from build123d import *

# Parameters (mm, degrees)
SKETCH1_W                                      = 222.53
SKETCH1_H                                      = 135
BOSS_EXTRUDE1_DEPTH                            = 6
FILLET1_R                                      = 5
CSK_FOR_M3_FLAT_HEAD_MACHINE_SCREW1_AT_2_COUNT = 2
CSK_FOR_M3_FLAT_HEAD_MACHINE_SCREW1_AT_2_PITCH = 211.53
CSK_FOR_M3_FLAT_HEAD_MACHINE_SCREW1_AT_3_COUNT = 2
CSK_FOR_M3_FLAT_HEAD_MACHINE_SCREW1_AT_3_PITCH = 245.195719579
CSK_FOR_M3_FLAT_HEAD_MACHINE_SCREW1_AT_4_COUNT = 2
CSK_FOR_M3_FLAT_HEAD_MACHINE_SCREW1_AT_4_PITCH = 124
CHAMFER1_SIZE                                  = 0.5
PCB_CUTOUT_DEPTH                               = 2
SKETCH8_W                                      = 20
SKETCH8_H                                      = 4.7
SKETCH8_W_2                                    = 16
SKETCH8_H_2                                    = 1.6
CABLE_RELIEF_DEPTH                             = 4.5
SKETCH9_W                                      = 25
SKETCH9_H                                      = 25
PI_CUTOUT_DEPTH                                = 3.2
USB_C_CUTOUT_REACH                             = 137
MOUSE_PAD_CUTOUT_DEPTH                         = 1.8
FILLET2_R                                      = 2


with BuildPart() as part:
    # Sketch1 → Boss-Extrude1 (new body)
    with BuildSketch(Plane(origin=(0, 0, 0), x_dir=(1, 0, 0), z_dir=(0, 1, 0))):
        with Locations((111.265, 67.5)):
            Rectangle(SKETCH1_W, SKETCH1_H)
    extrude(amount=BOSS_EXTRUDE1_DEPTH)

    # Fillet1
    fillet1_edges = [part.edges().sort_by_distance(p)[0] for p in [
        (0, 3, -135),
        (222.53, 3, -135),
        (222.53, 3, 0),
        (0, 3, 0),
    ]]
    fillet(fillet1_edges, radius=FILLET1_R)

    # Sketch4 → CSK for M3 Flat Head Machine Screw1 (revolve, cut)
    with BuildSketch(Plane(origin=(5.5, 0, -129.5), x_dir=(0, 0, -1), z_dir=(1, 0, 0))):
        Polygon((0, 0), (0, 6), (1.7, 6), (1.7, 2.95), (3.15, 1.5), (3.15, 0), align=None)
    csk_for_m3_flat_head_machine_screw1 = revolve(axis=Axis((5.5, -6.35, -129.5), (0, 1, 0)), mode=Mode.SUBTRACT)

    # CSK for M3 Flat Head Machine Screw1 at 2: CSK for M3 Flat Head Machine Screw1 ×2
    with Locations(*[(i * CSK_FOR_M3_FLAT_HEAD_MACHINE_SCREW1_AT_2_PITCH, 0, 0) for i in range(1, CSK_FOR_M3_FLAT_HEAD_MACHINE_SCREW1_AT_2_COUNT)]):
        add(csk_for_m3_flat_head_machine_screw1, mode=Mode.SUBTRACT)

    # CSK for M3 Flat Head Machine Screw1 at 3: CSK for M3 Flat Head Machine Screw1 ×2
    with Locations(*[Vector(0.862698584, 0, 0.505718453) * (i * CSK_FOR_M3_FLAT_HEAD_MACHINE_SCREW1_AT_3_PITCH) for i in range(1, CSK_FOR_M3_FLAT_HEAD_MACHINE_SCREW1_AT_3_COUNT)]):
        add(csk_for_m3_flat_head_machine_screw1, mode=Mode.SUBTRACT)

    # CSK for M3 Flat Head Machine Screw1 at 4: CSK for M3 Flat Head Machine Screw1 ×2
    with Locations(*[(0, 0, i * CSK_FOR_M3_FLAT_HEAD_MACHINE_SCREW1_AT_4_PITCH) for i in range(1, CSK_FOR_M3_FLAT_HEAD_MACHINE_SCREW1_AT_4_COUNT)]):
        add(csk_for_m3_flat_head_machine_screw1, mode=Mode.SUBTRACT)

    # Chamfer1
    chamfer1_edges = [part.edges().sort_by_distance(p)[0] for p in [
        (5.5, 0, -2.35),
        (217.03, 0, -2.35),
        (217.03, 0, -126.35),
        (5.5, 0, -126.35),
    ]]
    chamfer(chamfer1_edges, length=CHAMFER1_SIZE)

    # Sketch6 → PCB Cutout (cut)
    with BuildSketch(Plane(origin=(0, 6, 0), x_dir=(1, 0, 0), z_dir=(0, 1, 0))):
        with BuildLine():
            Line((12.5, 7.5), (210.03, 7.5))
            ThreePointArc((210.03, 7.5), (213.565533906, 8.964466094), (215.03, 12.5))
            Line((215.03, 12.5), (215.03, 122.5))
            ThreePointArc((215.03, 122.5), (213.565533906, 126.035533906), (210.03, 127.5))
            Line((210.03, 127.5), (12.5, 127.5))
            ThreePointArc((12.5, 127.5), (8.964466094, 126.035533906), (7.5, 122.5))
            Line((7.5, 122.5), (7.5, 12.5))
            ThreePointArc((7.5, 12.5), (8.964466094, 8.964466094), (12.5, 7.5))
        make_face()
    extrude(amount=-PCB_CUTOUT_DEPTH, mode=Mode.SUBTRACT)

    # Sketch8 → Cable Relief (cut)
    with BuildSketch(Plane(origin=(0, 6, 0), x_dir=(1, 0, 0), z_dir=(0, 1, 0))):
        with Locations((111.265, 132.65)):
            Rectangle(SKETCH8_W, SKETCH8_H)
        with Locations((111.265, 128.3)):
            Rectangle(SKETCH8_W_2, SKETCH8_H_2)
    extrude(amount=-CABLE_RELIEF_DEPTH, mode=Mode.SUBTRACT)

    # Sketch9 → Pi Cutout (cut)
    with BuildSketch(Plane(origin=(0, 4, 0), x_dir=(1, 0, 0), z_dir=(0, 1, 0))):
        with Locations((111.265, 115)):
            Rectangle(SKETCH9_W, SKETCH9_H)
    extrude(amount=-PI_CUTOUT_DEPTH, mode=Mode.SUBTRACT)

    # Sketch7 → USB C Cutout (cut, up to next)
    with BuildSketch(Plane(origin=(0, 0, -135), x_dir=(-1, 0, 0), z_dir=(0, 0, -1)), mode=Mode.PRIVATE) as usb_c_cutout_sk1:
        with BuildLine():
            Line((-114.265, 7.8), (-108.265, 7.8))
            ThreePointArc((-108.265, 7.8), (-107.204339828, 7.360660172), (-106.765, 6.3))
            Line((-106.765, 6.3), (-106.765, 5.5))
            ThreePointArc((-106.765, 5.5), (-107.204339828, 4.439339828), (-108.265, 4))
            Line((-108.265, 4), (-114.265, 4))
            ThreePointArc((-114.265, 4), (-115.325660172, 4.439339828), (-115.765, 5.5))
            Line((-115.765, 5.5), (-115.765, 6.3))
            ThreePointArc((-115.765, 6.3), (-115.325660172, 7.360660172), (-114.265, 7.8))
        make_face()
    usb_c_cutout_tool1 = extrude(usb_c_cutout_sk1.sketch, amount=-USB_C_CUTOUT_REACH, mode=Mode.PRIVATE) & part.part
    add(usb_c_cutout_tool1.solids().sort_by_distance((111.265, 5.9, -135))[0], mode=Mode.SUBTRACT)

    # Sketch5 → Mouse Pad Cutout (cut)
    with BuildSketch(Plane.XZ):
        Polygon((127.765, -126.035533906), (213.565533906, -126.035533906), (213.565533906, -8.964466094), (8.964466094, -8.964466094), (8.964466094, -126.035533906), (94.765, -126.035533906), (94.765, -99.035533906), (127.765, -99.035533906), align=None)
    extrude(amount=-MOUSE_PAD_CUTOUT_DEPTH, mode=Mode.SUBTRACT)

    # Fillet2
    fillet2_edges = [part.edges().sort_by_distance(p)[0] for p in [
        (101.265, 3.75, -135),
        (121.265, 3.75, -135),
    ]]
    fillet(fillet2_edges, radius=FILLET2_R)


solid = part.part
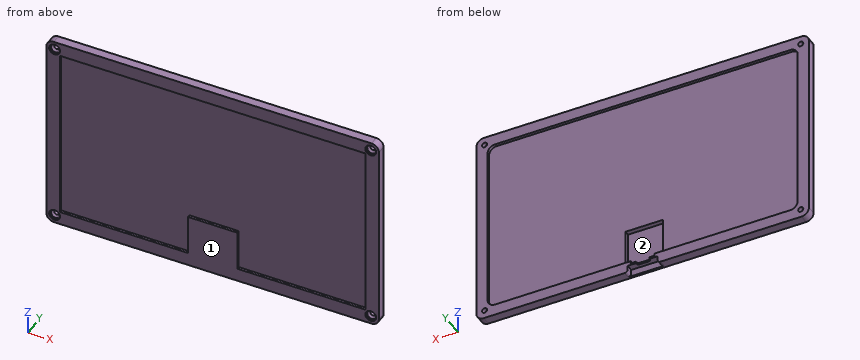
Design review of the part built by this model. Coordinates are the model's own, in mm. Face numbers are marked on the shaded views. Coordinates: 2 decimals unless noted, no trailing zeros. Order: outer loops, then holes, each group sorted by start corner. A loop starts at its lowest first (then second) coordinate and runs counter-clockwise, first axis right, second up. Notation, with made-up numbers: (33.25, 45.5) -> (74.25, 45.5) arc R15 ccw to (74.25, 65.5) -> close; hole circle Ø8 at (55.5, 75.5). An arc over 180 degrees is marked (long way). One line per item, written item: value.
1) To check wall thickness, follow probe 1 along X at (y, z) = (1.25, -129.5); probe 2 along X at (y, z) = (0.55, -106) (3 decimals); probe 3 along Z at (x, y) = (5.5, 1). State the ranges of each line that lie inside material, in increasing order. Write a range as [from, to].
Output values:
probe 1: x = [0, 2.35], [8.65, 213.88], [220.18, 222.53]
probe 2: x = [0, 8.964], [94.765, 127.765], [213.566, 222.53]
probe 3: z = [-135, -132.65], [-126.35, -8.65], [-2.35, 0]
2) We need section A-A, the plane x = 68. Give the boundary of the cut face in (y, z), then the cut area to 3 significant figures.
Output values:
outline: (0, -135) -> (6, -135) -> (6, -127.5) -> (4, -127.5) -> (4, -7.5) -> (6, -7.5) -> (6, 0) -> (0, 0) -> (0, -8.96) -> (1.8, -8.96) -> (1.8, -126.04) -> (0, -126.04) -> close
area: 359 mm2
3) We need section B-B, the plane z = -45. Give the boundary of the cut face in (x, y), then the cut area to 3 significant figures.
Output values:
outline: (0, 0) -> (8.96, 0) -> (8.96, 1.8) -> (213.57, 1.8) -> (213.57, 0) -> (222.53, 0) -> (222.53, 6) -> (215.03, 6) -> (215.03, 4) -> (7.5, 4) -> (7.5, 6) -> (0, 6) -> close
area: 552 mm2
4) Draft analysis for pull direction X (two halves, no side actions). For the marked faces 1 and 2, state which applies: +X half, -X half, draft (parallel to the pull), parting line (faces both ways), or undercut.
Output values:
face 1: draft
face 2: undercut
5) Clearance check with flat-ended pins moving along their axes: P1, Ø1.5, axis at x = 167.5, z = -68.5, coming from the +Y side; P2, Ø5, axis at x = 97.5, z = -95, coming from the -Y side. State where each tip first meets the part, or that it passes through.
Output values:
P1: stops at y = 4
P2: stops at y = 1.8
